from build123d import *

# Parameters (mm, degrees)
SKETCH_1_R          = 12.5
EXTRUDE_1_DEPTH     = 50
SKETCH_2_R          = 1.5
SKETCH_2_R_2        = 1.512365131
CUT_EXTRUDE_1_DEPTH = 10
SKETCH_3_R          = 2.5
EXTRUDE_2_DEPTH     = 20


with BuildPart() as part:
    # 草图1 → 凸台-拉伸1 (new body)
    with BuildSketch(Plane(origin=(0, 0, 0), x_dir=(1, 0, 0), z_dir=(0, 1, 0))):
        Circle(SKETCH_1_R)
    extrude(amount=EXTRUDE_1_DEPTH)

    # 草图2 → 切除-拉伸1 (cut)
    with BuildSketch(Plane(origin=(0, 50, 0), x_dir=(1, 0, 0), z_dir=(0, 1, 0))):
        with Locations((0, -10)):
            Circle(SKETCH_2_R)
        with Locations((0, 10)):
            Circle(SKETCH_2_R_2)
    extrude(amount=-CUT_EXTRUDE_1_DEPTH, mode=Mode.SUBTRACT)

    # 草图3 → 凸台-拉伸2 (add)
    with BuildSketch(Plane(origin=(0, 50, 0), x_dir=(1, 0, 0), z_dir=(0, 1, 0))):
        Circle(SKETCH_3_R)
    extrude(amount=EXTRUDE_2_DEPTH)


solid = part.part
The listing builds one solid part. Answer for the finished solid, in the listing's coordinates (mm). A direction names the side the tool comes from. Coordinates: 2 decimals unless noted, no trailing zeros. Loops run counter-clockwise (first coordinate to the right, second up) from the corner with the lowest first, then second, coordinate; pieces in that order, holes last. Notation, with made-up numbers: M 56,-20.5 L 69,-20.5 A20 cw 69,-0.5 Z; hole C 62.25,-18 d5. An arc over 180 degrees is marked long. Answer in a Markdown table with one row per item.
1) Determine the mould class of faces 3 (the flat face through (0, 50, 3)), 4 (the flat face through (0, 40, 10)), 5 (the cylindrical face through (-0.328, 45.07, -8.524)), 6 (the cylindrical face through (11.923, 24.65, -3.755)) for opening direction X: released by +X, released by -X, zero draft, split by the parting line, or undercut.
Answers below:
| item | result |
|---|---|
| face 3 | zero draft |
| face 4 | undercut |
| face 5 | undercut |
| face 6 | split by the parting line |
2) Find the intervals of material crossed by probe 1 along Z at (x, y) = (0, 43.25); probe 2 along Y at (x, z) = (9.5, 2); probe 3 along X at (y, z) = (42.75, 10), in increasing order.
Answers below:
| item | result |
|---|---|
| probe 1 | -12.5 to -11.51, -8.49 to 8.5, 11.5 to 12.5 |
| probe 2 | 0 to 50 |
| probe 3 | -7.5 to -1.5, 1.5 to 7.5 |
3) Find section A-A (z = 10). Determine the outline of the cut face in (x, y), then the cut area to 3 significant figures.
Answers below:
| item | result |
|---|---|
| outline | M -7.5,0 L 7.5,0 L 7.5,50 L 1.5,50 L 1.5,40 L -1.5,40 L -1.5,50 L -7.5,50 Z |
| area | 720 mm^2 |
4) Find section C-C (y = 41). Determine the outline of the cut face in (x, z).
Answers below:
| item | result |
|---|---|
| outline | C 0,0 d25; hole C 0,-10 d3.02; hole C 0,10 d3 |
5) Find section B-B (x = 0). Determine the outline of the cut face in (y, z).
Answers below:
| item | result |
|---|---|
| outline | M 0,-12.5 L 50,-12.5 L 50,-11.51 L 40,-11.51 L 40,-8.49 L 50,-8.49 L 50,-2.5 L 70,-2.5 L 70,2.5 L 50,2.5 L 50,8.5 L 40,8.5 L 40,11.5 L 50,11.5 L 50,12.5 L 0,12.5 Z |
6) Find section D-D (y = 59). Determine the outline of the cut face in (x, z).
Answers below:
| item | result |
|---|---|
| outline | C 0,0 d5 |
7) Which of the six approach directions +Z, -Z, +X, -X, +Y, -Y give full straight-line access (tool end or side, diameter ignored) to faces 1 (the cylindrical face through (-0.325, 45.07, 11.464)), 2 (the flat face through (0, 0, 0))?
Answers below:
| item | result |
|---|---|
| face 1 | +Y |
| face 2 | +Z, -Z, +X, -X, -Y |
8) Given pin 1 (2 mm diameter, centred on x = 0.5, z = 9.5, fed in from +Y); pin 2 (2.5 mm diameter, centred on x = 0, z = -10, fed in from +Y); pin 3 (6 mm diameter, centred on y = 37.5, z = 9, fed in from +X), each flat-ended and moving along its own axis, determine where each tip first touches the part or whether it passes through.
Answers below:
| item | result |
|---|---|
| pin 1 | y = 50 |
| pin 2 | y = 40 |
| pin 3 | x = 10.97 |
